For this review, take the finished solid that the model builds, in its own axes (mm). A direction names the side the tool comes from. Give positions to 0.01 mm unless a question says otherwise; leave off trailing zeros. Write each loop counter-clockwise with the first axis right and the second up, starting at its lowest first coordinate (ties: lowest second). Pieces come first, ordered by that corner, then holes.
Q1. For line 1 (X direction, y = -1.75, z = 0); line 2 (X direction, y = -1, z = -1); line 3 (Z direction, x = 147, y = 0.25), list the stretches that pass through material, from the lowest coordinate up.
Q2. We need section A-A (z = 0). Write out the cut boundary in (x, y) (3 decimals), then the cut area to 3 significant figures.
Q3. We need section D-D (x = 123). Write out the cut boundary in (y, z) (3 decimals), then the cut area to 3 significant figures.
Q4. Mouldability with a two-part tool opening along X and no side actions: class faces 3 (the flat face through (190.5, 0, 0)), 4 (the flat face through (50, 2.54, -1)), 5 (the flat face through (0, 0, 0)), 6 (the cylindrical face through (53.193, -0.359, -0.212)) as released by +X, released by -X, zero draft, split by the parting line, or undercut.
Q5. We need section C-C (x = 171.45). Write out the cut boundary in (y, z) (3 decimals).
Q6. Machinability: for faces 1 (the cylindrical face through (93.92, 0.14, 3.17)), 2 (the flat face through (170.7, 2.54, 1.7)), which of the approach directions +Z, -Z, +X, -X, +Y, -Y give a long, thin tool a straight path to every point of the face, cutting with its end or side? Answer none if there is none.
Q7. We need section B-B (y = 0). Write out the cut boundary in (x, z) (3 decimals), then the cut area to 3 significant figures.
Q8. Insertion check: P1, Ø0.5, axis at y = 3, z = 0, coming from the -X side; P2, Ø2, axis at x = 170.5, z = -1.5, coming from the +Y side. Each pin has a flat end and moves straight along its axis. Give the tip position at first contact, or say it passes through.
```python
from build123d import *

# Parameters (mm, degrees)
SKETCH1_R               = 3.175
BOSS_EXTRUDE1_DEPTH     = 190.5
CUT_EXTRUDE1_DEPTH      = 191.552909319
CUT_EXTRUDE1_DEPTH_BACK = 191.552909319
SKETCH2_R               = 1.63195
CUT_EXTRUDE2_START      = 2.54
SKETCH2_3_W             = 6.35
SKETCH2_3_H             = 14.521129012
SKETCH2_3_R             = 1.63195
SKETCH2_3_H_2           = 11.745313468
CUT_EXTRUDE2_DEPTH      = 189.012909422


with BuildPart() as part:
    # Sketch1 → Boss-Extrude1 (new body)
    with BuildSketch(Plane(origin=(0, 0, 0), x_dir=(0, 0, -1), z_dir=(1, 0, 0))):
        Circle(SKETCH1_R)
    extrude(amount=BOSS_EXTRUDE1_DEPTH)

    # Sketch2 → Cut-Extrude1 (cut, two sides: drawn at the far end of the back side and taken through both)
    with BuildSketch(Plane(origin=(0, 0, 0), x_dir=(1, 0, 0), z_dir=(0, 1, 0)).offset(-CUT_EXTRUDE1_DEPTH_BACK)):
        with Locations(Location((51.575, 0, 0), (0, 0, 270))):
            Circle(SKETCH2_R)
        with Locations(Location((69.075, 0, 0), (0, 0, 270))):
            Circle(SKETCH2_R)
        with Locations(Location((171.45, 0, 0), (0, 0, 270))):
            Circle(SKETCH2_R)
    extrude(amount=CUT_EXTRUDE1_DEPTH + CUT_EXTRUDE1_DEPTH_BACK, mode=Mode.SUBTRACT)

    # Sketch2_3 → Cut-Extrude2 (cut, through all)
    # profile 1 of 3: a face of its own
    with BuildSketch(Plane(origin=(0, 0, 0), x_dir=(1, 0, 0), z_dir=(0, 1, 0)).offset(CUT_EXTRUDE2_START)):
        with Locations((171.45, 0)):
            Rectangle(SKETCH2_3_W, SKETCH2_3_H)
        with Locations(Location((171.45, 0, 0), (0, 0, 270))):
            Circle(SKETCH2_3_R, mode=Mode.SUBTRACT)
    # profile 2 of 3: a face of its own
    with BuildSketch(Plane(origin=(0, 0, 0), x_dir=(1, 0, 0), z_dir=(0, 1, 0)).offset(CUT_EXTRUDE2_START)):
        with Locations((69.075, 0)):
            Rectangle(SKETCH2_3_W, SKETCH2_3_H_2)
        with Locations(Location((69.075, 0, 0), (0, 0, 270))):
            Circle(SKETCH2_3_R, mode=Mode.SUBTRACT)
    # profile 3 of 3: a face of its own
    with BuildSketch(Plane(origin=(0, 0, 0), x_dir=(1, 0, 0), z_dir=(0, 1, 0)).offset(CUT_EXTRUDE2_START)):
        with Locations((51.575, 0)):
            Rectangle(SKETCH2_3_W, SKETCH2_3_H_2)
        with Locations(Location((51.575, 0, 0), (0, 0, 270))):
            Circle(SKETCH2_3_R, mode=Mode.SUBTRACT)
    extrude(amount=CUT_EXTRUDE2_DEPTH, mode=Mode.SUBTRACT)


solid = part.part
```
Computed:
1. line 1: x = 0 to 49.94, 53.21 to 67.44, 70.71 to 169.82, 173.08 to 190.5
1. line 2: x = 0 to 50.29, 52.86 to 67.79, 70.36 to 170.16, 172.74 to 190.5
1. line 3: z = -3.17 to 3.17
2. outline: (0, -3.175) - (49.943, -3.175) - (49.943, 2.54) - (48.4, 2.54) - (48.4, 3.175) - (0, 3.175) - close; (53.207, -3.175) - (67.443, -3.175) - (67.443, 2.54) - (65.9, 2.54) - (65.9, 3.175) - (54.75, 3.175) - (54.75, 2.54) - (53.207, 2.54) - close; (70.707, -3.175) - (169.818, -3.175) - (169.818, 2.54) - (168.275, 2.54) - (168.275, 3.175) - (72.25, 3.175) - (72.25, 2.54) - (70.707, 2.54) - close; (173.082, -3.175) - (190.5, -3.175) - (190.5, 3.175) - (174.625, 3.175) - (174.625, 2.54) - (173.082, 2.54) - close
2. area: 1,140 mm2
3. outline: circle Ø6.35 at (0, 0)
3. area: 31.7 mm2
4. face 3: released by +X
4. face 4: undercut
4. face 5: released by -X
4. face 6: undercut
5. outline: (-2.723, -1.632) arc R3.175 ccw to (2.54, -1.905) - (2.54, -1.632) - close; (-2.723, 1.632) - (2.54, 1.632) - (2.54, 1.905) arc R3.175 ccw to start
6. face 1: +X, -X
6. face 2: +Z, -Z, +Y
7. outline: (0, -3.175) - (190.5, -3.175) - (190.5, 3.175) - (0, 3.175) - close; hole circle Ø3.264 at (51.575, 0); hole circle Ø3.264 at (69.075, 0); hole circle Ø3.264 at (171.45, 0)
7. area: 1,180 mm2
8. P1: stops at x = 0
8. P2: stops at y = 2.54
